For this review, take the finished solid that the model builds, in its own axes (mm). Face numbers are marked on the shaded views. A direction names the side the tool comes from. Round coordinates to 2 decimals unless told otherwise and drop trailing zeros. Loops run counter-clockwise (first coordinate to the right, second up) from the corner with the lowest first, then second, coordinate; pieces in that order, holes last.
1) Insertion check: pin 1 (7.5 mm diameter, centred on y = 10, z = 3.5, fed in from +X); pin 2 (2.5 mm diameter, centred on x = 15, z = -2.5, fed in from +Y). Each pin has a flat end and moves straight along its axis. Give the tip position at first contact, or say it passes through.
2) Tool access review of the marked faces 4 and 5: name each direction out of +Z, -Z, +X, -X, +Y, -Y from which nothing blocks a thin tool from reaching the whole face with its end or side.
3) Take a section at D-D (x = 15). Give the number of separate pieces and of enclosed holes in the cut face, then the cut area to 3 significant figures.
4) Take a section at A-A (x = 6). State the section outline as (y, z) points.
5) Take a section at C-C (y = 4.5). State the section outline as (x, z) points, then the cut area to 3 significant figures.
6) Wall thickness on L1, parallel to Z at x = 10.75, y = 4.5; L2, parallel to Z at x = 6, y = 6.5; L3, parallel to X at y = 7, z = -6: over which ranges is each line inside the solid? List them lowest first.
7) Take a section at B-B (z = -16). State the section outline as (x, y) points, then the cut area to 3 significant figures.
8) Mouldability with a two-part tool opening along X and no side actions: class the marked faces 1, 2 and 3 as pulls with the +X half, pulls with the -X half, needs draft (parallel to the pull), parting line crosses it, or undercut.
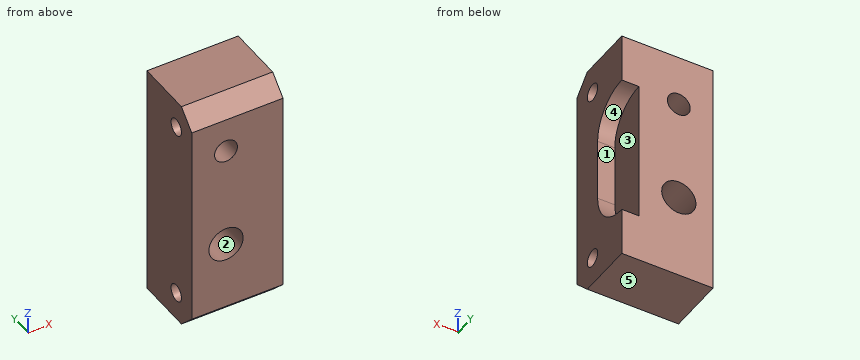
Autodesk Inventor part; units mm, degrees
ref_plane "YZ Plane" through (0, 0, 0) normal (1, 0, 0) x (0, 1, 0)
ref_plane "XZ Plane" through (0, 0, 0) normal (0, 1, 0) x (-1, 0, 0)
ref_plane "XY Plane" through (0, 0, 0) normal (0, 0, 1) x (1, 0, 0)
sketch "Szkic1" plane through (0, 0, 0) normal (1, 0, 0) x (0, 1, 0)
  line L0 (13, 21) -> (0, 21)
  line L1 (0, 21) -> (0, -21)
  line L2 (0, -21) -> (13, -21)
  line L3 (13, -21) -> (13, 21)
  line L4 (0, 0) -> (13, 0) construction
  dimension "d0" = 42
  dimension "d1" = 13
extrude "Wyciągnięcie proste3" add sketch "Szkic1" along normal blind 16
sketch "Szkic4" plane through (16, 0, 0) normal (1, 0, 0) x (0, 0, -1)
  line L0 (-12.5, 13) -> (12.5, 13)
  line L1 (12.5, 13) -> (12.5, 6)
  line L2 (12.5, 6) -> (-12.5, 6)
  line L3 (-12.5, 6) -> (-12.5, 13)
  line L4 (0, 6) -> (0, 0) construction
  line L5 (21, 13) -> (-21, 13)
  point P0 (0, 13)
  dimension "d10" = 25
  dimension "d11" = 7
extrude "Wyciągnięcie proste4" cut sketch "Szkic4" against normal blind 3
fillet "Zaokrąglenie1" radius 7 2 edges at (14.5, 6, 12.5) (14.5, 6, -12.5)
sketch "Szkic5" plane through (16, 0, 0) normal (1, 0, 0) x (0, 0, -1)
  line L0 (0, 0) -> (0, 13) construction
  line L1 (-12.5, 13) -> (12.5, 13)
  line L2 (-21, 13) -> (-21, 0)
  line L3 (-21, 0) -> (21, 0)
  point P0 (-16, 4.5)
  point P1 (16, 4.5)
  dimension "d15" = 32
  dimension "d17" = 4.5
hole "Otwór1" at (16, 4.5, 16) at (16, 4.5, -16) direction (-1, 0, 0) diameter 3 end through all
chamfer "Faza1" distance 3 angle 45 2 edges at (8, 0, 21) (8, 0, -21)
sketch "Szkic6" plane through (0, 0, -18) normal (0, -1, 0) x (1, 0, 0)
  line L0 (0, -3) -> (16, -3)
  line L1 (0, 36) -> (0, 0)
  point P0 (0, 18)
  point P1 (6, 12)
  dimension "d28" = 15
  dimension "d29" = 6
hole "Otwór2" at (6, 0, -6) direction (0, 1, 0) diameter 6 end through all
sketch "Szkic7" plane through (0, 0, -18) normal (0, -1, 0) x (1, 0, 0)
  line L0 (16, 39) -> (0, 39)
  circle A0 centre (6, 12) radius 3
  point P0 (0, 18)
  point P1 (6, 30)
  dimension "d37" = 9
hole "Otwór3" at (6, 0, 12) direction (0, 1, 0) diameter 4 end through all
thread "Gwint1"
thread "Gwint2"
thread "Gwint3"
thread "Gwint4"
properties part number "33_ekstruder1"
Response:
1. pin 1: stops at x = 13
1. pin 2: stops at y = 6
2. face 4: +X, +Y
2. face 5: -Z, +X, -X, +Y, -Y
3. separate pieces: 1
3. enclosed holes: 2
3. area: 369 mm2
4. outline: (0, -18) - (3, -21) - (13, -21) - (13, -9) - (0, -9) - close; (0, -3) - (13, -3) - (13, 10) - (0, 10) - close; (0, 14) - (13, 14) - (13, 21) - (3, 21) - (0, 18) - close; hole circle Ø3 at (4.5, -16); hole circle Ø3 at (4.5, 16)
5. outline: (0, -21) - (16, -21) - (16, -17.5) - (0, -17.5) - close; (0, -14.5) - (16, -14.5) - (16, 14.5) - (0, 14.5) - close; (0, 17.5) - (16, 17.5) - (16, 21) - (0, 21) - close; hole circle Ø6 at (6, -6); hole circle Ø4 at (6, 12)
5. area: 535 mm2
6. L1: z = -21 to -17.5, -14.5 to 14.5, 17.5 to 21
6. L2: z = -21 to -9, -3 to 10, 14 to 21
6. L3: x = 0 to 3, 9 to 13
7. outline: (0, 0) - (16, 0) - (16, 3) - (0, 3) - close; (0, 6) - (16, 6) - (16, 13) - (0, 13) - close
7. area: 160 mm2
8. face 1: needs draft
8. face 2: undercut
8. face 3: pulls with the +X half
